For this review, use the dimensioned drawing (mm, ordinates from the lowest corner) and the shaded views. Give positions to 0.01 mm unless a question says otherwise; leave off trailing zeros. Write each loop counter-clockwise with the first axis right and the second up, starting at its lowest first coordinate (ties: lowest second). Pieces come first, ordered by that corner, then holes. Notation, with made-up numbers: (-6, 73) -> (13, 73) arc R15 ccw to (13, 81) -> close; hole circle Ø9 at (2, 27.25). An arc over 180 degrees is marked (long way). Answer as CSV lines item,"result".
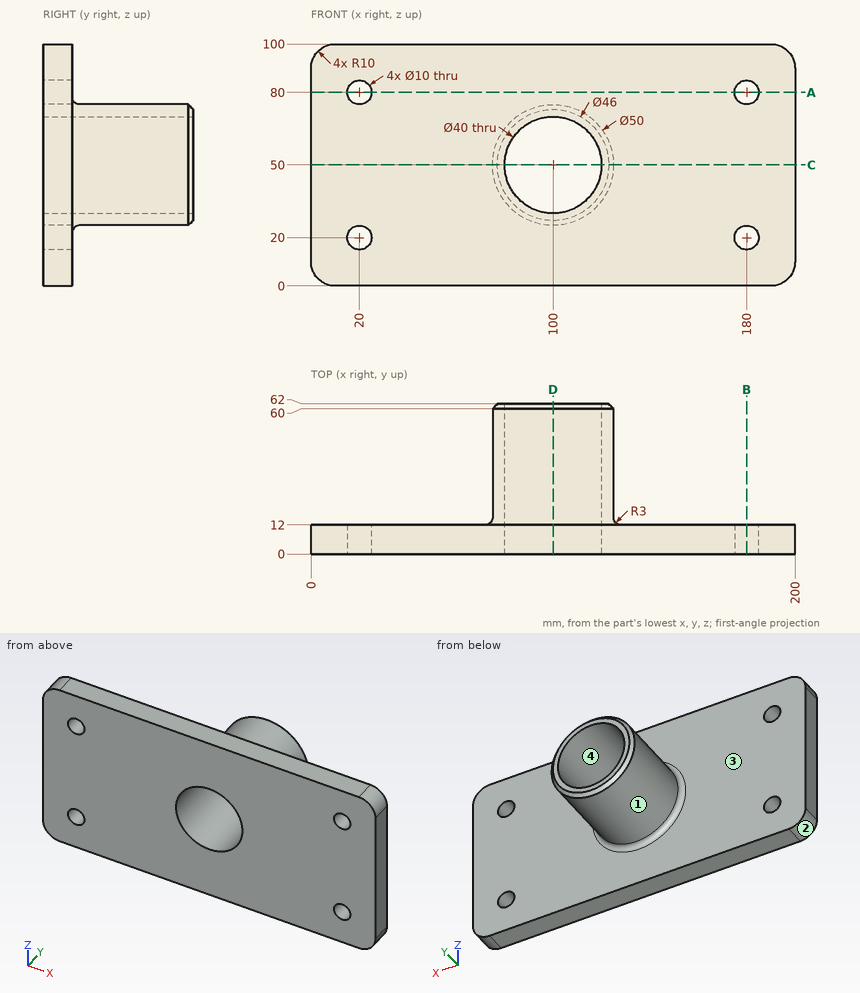
Q1. Add section D-D (x = 100). Write out the cut boundary in (y, z), plus the area to 3 significant figures.
Answer block:
outline,"(0, 0) -> (12, 0) -> (12, 22) arc R3 cw to (15, 25) -> (60, 25) -> (62, 27) -> (62, 30) -> (0, 30) -> close; (0, 70) -> (62, 70) -> (62, 73) -> (60, 75) -> (15, 75) arc R3 cw to (12, 78) -> (12, 100) -> (0, 100) -> close"
area,"1,220 mm2"
Q2. Clearance check with flat-ended pins moving along their axes: pin 1 (4 mm diameter, centred on x = 148.5, z = 59.5, fed in from +Y); pin 2 (5 mm diameter, centred on y = 40.5, z = 65, fed in from +X); pin 3 (4 mm diameter, centred on y = 33, z = 68, fed in from +X). State where each tip first meets the part, or that it passes through.
Answer block:
pin 1,"stops at y = 12"
pin 2,"stops at x = 121.65"
pin 3,"stops at x = 119.21"
Q3. Add section A-A (z = 80). Write out the cut boundary in (x, y), plus the area to 3 significant figures.
Answer block:
outline,"(0, 0) -> (15, 0) -> (15, 12) -> (0, 12) -> close; (25, 0) -> (175, 0) -> (175, 12) -> (25, 12) -> close; (185, 0) -> (200, 0) -> (200, 12) -> (185, 12) -> close"
area,"2,160 mm2"
Q4. Add section B-B (x = 180). Write out the cut boundary in (y, z).
Answer block:
outline,"(0, 0) -> (12, 0) -> (12, 15) -> (0, 15) -> close; (0, 25) -> (12, 25) -> (12, 75) -> (0, 75) -> close; (0, 85) -> (12, 85) -> (12, 100) -> (0, 100) -> close"
Q5. Draft analysis for pull direction X (two halves, no side actions). For the marked faces 1, 2, 3 and 4, state which applies: released by +X, released by -X, zero draft, split by the parting line, or undercut.
Answer block:
face 1,"split by the parting line"
face 2,"released by -X"
face 3,"zero draft"
face 4,"undercut"
Q6. To check wall thickness, follow probe 1 along Z at (x, y) = (20, 7.75); probe 2 along X at (y, z) = (3, 80); probe 3 along Z at (x, y) = (182.5, 5). State the ranges of each line that lie inside material, in increasing order. Write a range as [from, to].
Answer block:
probe 1,"z = [0, 15], [25, 75], [85, 100]"
probe 2,"x = [0, 15], [25, 175], [185, 200]"
probe 3,"z = [0, 15.67], [24.33, 75.67], [84.33, 100]"
Q7. Add section C-C (z = 50). Write out the cut boundary in (x, y), plus the area to 3 significant figures.
Answer block:
outline,"(0, 0) -> (80, 0) -> (80, 62) -> (77, 62) -> (75, 60) -> (75, 15) arc R3 cw to (72, 12) -> (0, 12) -> close; (120, 0) -> (200, 0) -> (200, 12) -> (128, 12) arc R3 cw to (125, 15) -> (125, 60) -> (123, 62) -> (120, 62) -> close"
area,"2,420 mm2"
